```python
from build123d import *

# Parameters (mm, degrees)
F1_DEPTH  = 15
F2_DEPTH  = 12.5
F4_DEPTH  = 5
F5_W      = 5
F5_H      = 2.5
F6_DEPTH  = 50
F7_W      = 5
F7_H      = 2.5
F8_DEPTH  = 5
F9_W      = 5
F9_H      = 2.5
F10_DEPTH = 5
F11_DEPTH = 10


with BuildPart() as f1:
    # F0 (on Top) → F1 (new body)
    with BuildSketch(Plane.XY):
        with BuildLine():
            ThreePointArc((46.1134053767, -25), (21.1134053767, 0), (46.1134053767, 25))
            Line((46.1134053767, 25), (46.1134053767, 30))
            Line((46.1134053767, 30), (21.1134053767, 30))
            Line((21.1134053767, 30), (-3.8865946233, 20))
            Line((-3.8865946233, 20), (-71.3865946233, 20))
            Line((-71.3865946233, 20), (-71.3865946233, -20))
            Line((-71.3865946233, -20), (-3.8865946233, -20))
            Line((-3.8865946233, -20), (21.1134053767, -30))
            Line((21.1134053767, -30), (46.1134053767, -30))
            Line((46.1134053767, -30), (46.1134053767, -25))
        make_face()
        Polygon((-63.8865946233, 12.5), (-63.8865946233, 0), (-63.8865946233, -12.5), (-68.8865946233, -12.5), (-68.8865946233, 12.5), align=None, mode=Mode.SUBTRACT)
        Polygon((-53.8865946233, 12.5), (-53.8865946233, 0), (-53.8865946233, -12.5), (-58.8865946233, -12.5), (-58.8865946233, 12.5), align=None, mode=Mode.SUBTRACT)
        Polygon((-43.8865946233, 12.5), (-43.8865946233, 0), (-43.8865946233, -12.5), (-48.8865946233, -12.5), (-48.8865946233, 12.5), align=None, mode=Mode.SUBTRACT)
        Polygon((-33.8865946233, 12.5), (-33.8865946233, 0), (-33.8865946233, -12.5), (-38.8865946233, -12.5), (-38.8865946233, 12.5), align=None, mode=Mode.SUBTRACT)
        Polygon((-23.8865946233, 12.5), (-23.8865946233, 0), (-23.8865946233, -12.5), (-28.8865946233, -12.5), (-28.8865946233, 12.5), align=None, mode=Mode.SUBTRACT)
        Polygon((-13.8865946233, 12.5), (-13.8865946233, 0), (-13.8865946233, -12.5), (-18.8865946233, -12.5), (-18.8865946233, 12.5), align=None, mode=Mode.SUBTRACT)
        Polygon((11.1134053767, 2.5), (11.1134053767, 0), (11.1134053767, -2.5), (6.1134053767, -2.5), (6.1134053767, 2.5), align=None, mode=Mode.SUBTRACT)
    extrude(amount=F1_DEPTH)

    # F2 (add): a face of the model
    f2_faces = [f1.faces().sort_by_distance(p)[0] for p in [
        (-71.3865946233, 0, 7.5),
    ]]
    extrude(f2_faces, amount=F2_DEPTH)

    # F3 (on face) → F4 (join)
    with BuildSketch(Plane(origin=(-83.8865946233, 0, 0), x_dir=(0, -1, 0), z_dir=(-1, 0, 0))):
        with BuildLine():
            ThreePointArc((-5.2915026221, 15), (-3.2915026221, 1.7084973779), (8, 9))
            ThreePointArc((8, 9), (7.2915026221, 12.2915026221), (5.2915026221, 15))
            Line((5.2915026221, 15), (-5.2915026221, 15))
        make_face()
        with BuildLine():
            Line((-5.2915026221, 15), (5.2915026221, 15))
            ThreePointArc((5.2915026221, 15), (0, 17), (-5.2915026221, 15))
        make_face()
    extrude(amount=F4_DEPTH)

    # F5 (on face) → F6 (cut)
    with BuildSketch(Plane.XZ.offset(20)):
        with Locations((-6.3865946233, 6.25)):
            Rectangle(F5_W, F5_H)
        with Locations((-6.3865946233, 8.75)):
            Rectangle(F5_W, F5_H)
    extrude(amount=-F6_DEPTH, mode=Mode.SUBTRACT)

    # F7 (on face) → F8 (cut)
    with BuildSketch(Plane.XZ.offset(20)):
        with Locations((-21.3865946233, 8.75)):
            Rectangle(F7_W, F7_H)
        with Locations((-21.3865946233, 6.25)):
            Rectangle(F7_W, F7_H)
    extrude(amount=-F8_DEPTH, mode=Mode.SUBTRACT)

    # F9 (on face) → F10 (cut)
    with BuildSketch(Plane(origin=(0, 20, 0), x_dir=(-1, 0, 0), z_dir=(0, 1, 0))):
        with Locations((21.3865946233, 8.75)):
            Rectangle(F9_W, F9_H)
        with Locations((21.3865946233, 6.25)):
            Rectangle(F9_W, F9_H)
    extrude(amount=-F10_DEPTH, mode=Mode.SUBTRACT)

    # F0 (on Top) → F11 (join)
    with BuildSketch(Plane.XY):
        Polygon((-63.8865946233, -12.5), (-63.8865946233, 0), (-63.8865946233, 12.5), (-68.8865946233, 12.5), (-68.8865946233, -12.5), align=None)
        Polygon((-53.8865946233, -12.5), (-53.8865946233, 0), (-53.8865946233, 12.5), (-58.8865946233, 12.5), (-58.8865946233, -12.5), align=None)
        Polygon((-43.8865946233, -12.5), (-43.8865946233, 0), (-43.8865946233, 12.5), (-48.8865946233, 12.5), (-48.8865946233, -12.5), align=None)
        Polygon((-33.8865946233, -12.5), (-33.8865946233, 0), (-33.8865946233, 12.5), (-38.8865946233, 12.5), (-38.8865946233, -12.5), align=None)
        Polygon((-23.8865946233, -12.5), (-23.8865946233, 0), (-23.8865946233, 12.5), (-28.8865946233, 12.5), (-28.8865946233, -12.5), align=None)
        Polygon((-13.8865946233, -12.5), (-13.8865946233, 0), (-13.8865946233, 12.5), (-18.8865946233, 12.5), (-18.8865946233, -12.5), align=None)
        Polygon((11.1134053767, -2.5), (11.1134053767, 0), (11.1134053767, 2.5), (6.1134053767, 2.5), (6.1134053767, -2.5), align=None)
    extrude(amount=F11_DEPTH)


solid = f1.part
```
For this review, take the finished solid that the model builds, in its own axes (mm). A direction names the side the tool comes from. Round coordinates to 2 decimals unless told otherwise and drop trailing zeros. Write each loop counter-clockwise with the first axis right and the second up, starting at its lowest first coordinate (ties: lowest second). Pieces come first, ordered by that corner, then holes. Notation, with made-up numbers: (-33, -2.75) - (16, -2.75) arc R5 ccw to (16, 4.25) - close; hole circle Ø5 at (-10, 85.5). An arc over 180 degrees is marked (long way). Write each question's results on one line, items separated by ' | '.
Item 1: Take a section at A-A on x = -25.5. State the section outline as (y, z) points, then the cut area to 3 significant figures.
Calculated:
outline: (-20, 0) - (20, 0) - (20, 15) - (12.5, 15) - (12.5, 10) - (-12.5, 10) - (-12.5, 15) - (-20, 15) - close | area: 475 mm^2
Item 2: For pin 1 (5 mm diameter, centred on x = -14.5, z = 8.5, fed in from +Y); pin 2 (5.5 mm diameter, centred on x = -57, y = 0, fed in from +Z); pin 3 (5 mm diameter, centred on y = -2.5, z = 10.5, fed in from +X), all flat-tipped, find the tip position at first contact; note any pin that passes through.
Calculated:
pin 1: stops at y = 20 | pin 2: stops at z = 15 | pin 3: stops at x = 21.62
Item 3: Take a section at C-C on z = 11.75. Count the separate pieces of the cut face and the enclosed holes in it, then the cut area to 3 significant figures.
Calculated:
separate pieces: 1 | enclosed holes: 7 | area: 4,270 mm^2
Item 4: Draft analysis for pull direction Z (two halves, no side actions). For faces 6 (the face through (-66, 0, 10)), 7 (the face through (-6, 0, 5)), 8 (the face through (-43, 20, 7)), state which applies: pulls with the +Z half, pulls with the -Z half, needs draft (parallel to the pull), parting line crosses it, or undercut.
Calculated:
face 6: pulls with the +Z half | face 7: undercut | face 8: needs draft
Item 5: For faces 1 (the face through (21.12, -0.55, 7.4)), 2 (the face through (-23.887, -18, 8)), 3 (the face through (-6, 0, 10)), 4 (the face through (-18.887, 18, 8)), 5 (the face through (-26, 12.5, 12)), list the 3-axis set-ups (+Z, -Z, +X, -X, +Y, -Y) from which the entire face can be reached by the end or side of a thin tool; tool diameter is ignored.
Calculated:
face 1: +Z, -Z, +X | face 2: -Y | face 3: +Y, -Y | face 4: +Y | face 5: +Z
Item 6: Take a section at D-D on y = 22. State the section outline as (x, z) points, then the cut area to 3 significant figures.
Calculated:
outline: (1.11, 0) - (34.24, 0) - (34.24, 15) - (1.11, 15) - close | area: 497 mm^2
Item 7: To check wall thickness, follow line 1 along Y through (x, z) = (-55.5, 10.5); line 2 along X through (y, z) = (-15.5, 9.25); line 3 along Y through (x, z) = (-30.5, 5). State the ranges of each line that lie inside material, in increasing order. Write a range as from..to.
Calculated:
line 1: y = -20..-12.5, 12.5..20 | line 2: x = -83.89..-23.89, -18.89..-8.89, -3.89..26.5 | line 3: y = -20..20
Item 8: Take a section at B-B on z = 2.5. State the section outline as (x, y) points, then the cut area to 3 significant figures.
Calculated:
outline: (-88.89, -4.66) - (-83.89, -4.66) - (-83.89, -20) - (-3.89, -20) - (21.11, -30) - (46.11, -30) - (46.11, -25) arc R25 cw to (46.11, 25) - (46.11, 30) - (21.11, 30) - (-3.89, 20) - (-83.89, 20) - (-83.89, 4.66) - (-88.89, 4.66) - close | area: 5,010 mm^2
